```python
from build123d import *

# Parameters (mm, degrees)
F0_R     = 5
F0_R_2   = 100
F1_DEPTH = 10


# Not quite as in the source:
# - ends of sketch curves that miss each other by under 0.0002 mm in the source are joined


with BuildPart() as f1:
    # F0 (on Front) → F1 (new body)
    with BuildSketch(Plane.XZ):
        with BuildLine():
            add(Edge.make_bspline(
                [(169.1493929479, -45.6158926146), (159.7651292122, -107.4219847214), (22.7183427382, -273.4801182779), (-224.8579575674, -226.7328438), (-267.6564696794, -202.0572125126)],
                knots=[0, 0, 0, 0, 0.4871765071, 1, 1, 1, 1], degree=3))
            ThreePointArc((169.1493929479, -45.6158926146), (-35.404456431, 171.5122555076), (-136.3616027906, -109.1914398753))
            add(Edge.make_bspline(
                [(-229.8119745952, -132.8222825671), (-188.6496121839, -169.4869168537), (-99.4743329729, -150.4504772299), (-136.3616027906, -109.1914398753)],
                knots=[0, 0, 0, 0, 96.391849846, 96.391849846, 96.391849846, 96.391849846], degree=3))
            ThreePointArc((-229.8119745952, -132.8222825671), (-289.6255876831, -145.0881241092), (-267.6564696794, -202.0572125126))
        make_face()
        with Locations((-254.5268251568, -164.2734536378)):
            Circle(F0_R, mode=Mode.SUBTRACT)
        with BuildLine():
            ThreePointArc((-96.6455557461, 97.0129985964), (-136.73540255, 0.1825598604), (-96.6455557461, -96.6478788756))
            ThreePointArc((-96.6455557461, -96.6478788756), (-96.6478779601, -103.7189453909), (-103.7189453903, -103.7166222615))
            ThreePointArc((-103.7189453903, -103.7166222615), (-146.7353999615, 0.1825598604), (-103.7189444749, 104.0817410675))
            ThreePointArc((-103.7189444749, 104.0817410675), (-96.6478779601, 104.0840651118), (-96.6455557461, 97.0129985964))
        make_face(mode=Mode.SUBTRACT)
        with Locations((0.2485292707, 0.1825598604)):
            Circle(F0_R_2, mode=Mode.SUBTRACT)
        with BuildLine():
            ThreePointArc((96.6478838863, -96.2804310179), (136.6228090286, 0.1825598604), (96.6478838863, 96.6455507387))
            ThreePointArc((96.6478838863, 96.6455507387), (96.6455499466, 103.7166173731), (103.7166173736, 103.7189505206))
            ThreePointArc((103.7166173736, 103.7189505206), (146.6228067875, 0.1825598604), (103.7166165815, -103.3538300071))
            ThreePointArc((103.7166165815, -103.3538300071), (96.6455499466, -103.3514976522), (96.6478838863, -96.2804310179))
        make_face(mode=Mode.SUBTRACT)
    extrude(amount=F1_DEPTH)


solid = f1.part
```
Source: CAD feature listing. Evaluate the final solid. Frame: model axes, mm. A direction names the side the tool comes from. Coordinates: 2 decimals unless noted, no trailing zeros. Loops run counter-clockwise (first coordinate to the right, second up) from the corner with the lowest first, then second, coordinate; pieces in that order, holes last. Notation, with made-up numbers: M 71.25,9 L 90.25,9 A9 cw 90.25,20 Z; hole C 81.5,-15.75 d3. An arc over 180 degrees is marked long. Use a Markdown table: item, result. Add a question column.
Q1. Material intervals for L1, parallel to X at y = -4, z = 1; L2, parallel to X at y = -7.75, z = 90; L3, parallel to Z at x = -62, y = -3.5, sorted ascending.
Q2. Section query B-B, the plane z = 84.5. Return loops of the section in (x, y).
Q3. Section query A-A, the plane z = -26. Return loops of the section in (x, y), and give its area (3 significant figures).
Q4. First-contact query: pin 1 (3 mm diameter, centred on y = -4.5, z = -190, fed in from +X); pin 2 (1.5 mm diameter, centred on y = -5, z = -33.5, fed in from +X); pin 3 (2 mm diameter, centred on x = -151.5, y = -8, fed in from -Z). Flat tips, straight axial feed; report the tip coordinate or a pass-through.
Q5. Section query D-D, the plane z = 131.5. Return loops of the section in (x, y).
Q6. Section query C-C, the plane y = -1.75. State how many separate pieces and enclosed holes the cut face has, and give its area (3 significant figures).
Q7. Draft query along Z for faces 1 (the flat face through (-56, -10, -96)), 2 (the cylindrical face through (136.615, -4.93, -1.318)), 3 (the cylindrical face through (-289.15, -4.93, -144.24)). Return one class per face: pulls with the +Z half, pulls with the -Z half, needs draft (parallel to the pull), parting line crosses it, or undercut.
Q8. Access query for faces 4 (the flat face through (-56, 0, -96)), 5 (the cylindrical face through (-146.727, -4.93, -1.433)). Directions: +Z, -Z, +X, -X, +Y, -Y. A direction counts if a zero-diameter tool reaches every point of the face in a straight line with its end or side. Return the directions, or none.
Result:
| question | item | result |
|---|---|---|
| 1 | L1 | x = -174.75 to -146.73, -136.73 to -99.75, 100.25 to 136.62, 146.62 to 175.25 |
| 1 | L2 | x = -149.94 to -116.1, -103.18 to -43.72, 44.21 to 102.87, 115.83 to 150.44 |
| 1 | L3 | z = -231.71 to -78.08, 78.45 to 163.74 |
| 2 | outline | M -153.1,-10 L -120.15,-10 L -120.15,0 L -153.1,0 Z; M -107.71,-10 L -53.52,-10 L -53.52,0 L -107.71,0 Z; M 54.01,-10 L 107.43,-10 L 107.43,0 L 54.01,0 Z; M 119.9,-10 L 153.6,-10 L 153.6,0 L 119.9,0 Z |
| 3 | outline | M -172.78,-10 L -144.38,-10 L -144.38,0 L -172.78,0 Z; M -134.21,-10 L -96.26,-10 L -96.26,0 L -134.21,0 Z; M 96.76,-10 L 134.09,-10 L 134.09,0 L 96.76,0 Z; M 144.26,-10 L 173.28,-10 L 173.28,0 L 144.26,0 Z |
| 3 | area | 1,330 mm2 |
| 4 | pin 1 | stops at x = 62.87 |
| 4 | pin 2 | stops at x = 172.12 |
| 4 | pin 3 | stops at z = -232.03 |
| 5 | outline | M -115.43,-10 L 115.92,-10 L 115.92,0 L -115.43,0 Z |
| 6 | separate pieces | 1 |
| 6 | enclosed holes | 4 |
| 6 | area | 85,900 mm2 |
| 7 | face 1 | needs draft |
| 7 | face 2 | undercut |
| 7 | face 3 | parting line crosses it |
| 8 | face 4 | +Z, -Z, +X, -X, +Y |
| 8 | face 5 | +Y, -Y |
